from build123d import *

# Parameters (mm, degrees)
BOSS_EXTRUDE1_DEPTH = 14.2
BOSS_EXTRUDE2_DEPTH = 2.8
SKETCH3_R           = 1.7
CUT_EXTRUDE2_DEPTH  = 70.686512325


with BuildPart() as part:
    # Sketch1 → Boss-Extrude1 (new body)
    with BuildSketch(Plane(origin=(0, 0, 0), x_dir=(1, 0, 0), z_dir=(0, 1, 0))):
        Polygon((0, 21.05), (0, 31.1), (50, 31.1), (50, 21.05), (58, 21.05), (58, 10.05), (50, 10.05), (50, 0), (0, 0), (0, 10.05), (-8, 10.05), (-8, 21.05), align=None)
    extrude(amount=BOSS_EXTRUDE1_DEPTH)

    # Sketch2 → Boss-Extrude2 (add)
    with BuildSketch(Plane(origin=(0, 14.2, 0), x_dir=(1, 0, 0), z_dir=(0, 1, 0))):
        with BuildLine():
            Line((57.5, 31.1), (-7.5, 31.1))
            ThreePointArc((-7.5, 31.1), (-9.267766953, 30.367766953), (-10, 28.6))
            Line((-10, 28.6), (-10, 2.5))
            ThreePointArc((-10, 2.5), (-9.267766953, 0.732233047), (-7.5, 0))
            Line((-7.5, 0), (57.5, 0))
            ThreePointArc((57.5, 0), (59.267766953, 0.732233047), (60, 2.5))
            Line((60, 2.5), (60, 28.6))
            ThreePointArc((60, 28.6), (59.267766953, 30.367766953), (57.5, 31.1))
        make_face()
    extrude(amount=BOSS_EXTRUDE2_DEPTH)

    # Sketch3 → Cut-Extrude2 (cut, through all)
    with BuildSketch(Plane(origin=(0, 17, 0), x_dir=(1, 0, 0), z_dir=(0, 1, 0))):
        with Locations(Location((-6.8, 3.2, 0), (0, 0, 270))):
            Circle(SKETCH3_R)
        with Locations(Location((56.8, 3.2, 0), (0, 0, 270))):
            Circle(SKETCH3_R)
        with Locations(Location((56.8, 27.9, 0), (0, 0, 270))):
            Circle(SKETCH3_R)
        with Locations(Location((-6.8, 27.9, 0), (0, 0, 270))):
            Circle(SKETCH3_R)
    extrude(amount=-CUT_EXTRUDE2_DEPTH, mode=Mode.SUBTRACT)


solid = part.part
Work out the finished part from the listing and answer in its coordinate system (mm). A direction names the side the tool comes from. Give positions to 0.01 mm unless a question says otherwise; leave off trailing zeros. Order: outer loops, then holes, each group sorted by start corner. A loop starts at its lowest first (then second) coordinate and runs counter-clockwise, first axis right, second up. Notation, with made-up numbers: (22.25, 14.25) - (27.25, 14.25) arc R23 ccw to (27.25, 38.25) - close; hole circle Ø8 at (15, 45). An arc over 180 degrees is marked (long way). Answer as CSV lines item,"result". Start each with the question number.
Q1. Find the intervals of material crossed by L1, parallel to X at y = 16.4, z = -27.9; L2, parallel to X at y = 5, z = -2; L3, parallel to X at y = 14.25, z = -28.5, in increasing order. Write a range as [from, to].
Q2. For faces 1 (the face through (50, 7, -26)), 2 (the face through (0, 7, -5)), 3 (the face through (50, 7, -5)), 4 (the face through (-4, 7, -21.05)), determine the directions among +Z, -Z, +X, -X, +Y, -Y from which every point of the face is accessible in a straight line to the end or side of a thin tool.
Q3. The mould has two halves that part along Z. Classify faces 5 (the face through (59.287, 15.58, -30.348)), 6 (the face through (25, 8, 0)), 7 (the face through (-5.65, 15.62, -4.45)): +Z half, -Z half, draft (parallel to the pull), parting line (faces both ways), or undercut.
Q4. The part is cut by section B-B (z = -3.2). Write down the section's boundary in (x, y), then the cut area to 3 significant figures.
Q5. The part is cut by section C-C (y = 1.25). Write down the section's boundary in (x, z), then the cut area to 3 significant figures.
Q6. The part is cut by section D-D (z = -22). Write down the section's boundary in (x, y).
Q7. The part is cut by section A-A (x = -6.8). Write down the section's boundary in (y, z).
Q8. Given pin 1 Ø5 at (y, z) = (5, -3) entering from -X; pin 2 Ø5.5 at (y, z) = (7, -14) entering from -X; pin 3 Ø9 at (y, z) = (9.5, -16) entering from +X; pin 4 Ø2 at (x, z) = (-6.8, -27.9) entering from -Y, each flat-ended and moving along its own axis, determine where each tip first touches the part or whether it passes through.
Check result:
1,L1,"x = [-10, -8.5], [-5.1, 55.1], [58.5, 60]"
1,L2,"x = [0, 50]"
1,L3,"x = [-10, -8.39], [-5.21, 55.21], [58.39, 60]"
2,face 1,"-Z, +X, -Y"
2,face 2,"+Z, -X, -Y"
2,face 3,"+Z, +X, -Y"
2,face 4,"-Z, -X, -Y"
3,face 5,"-Z half"
3,face 6,"+Z half"
3,face 7,"undercut"
4,outline,"(-10, 14.2) - (-8.5, 14.2) - (-8.5, 17) - (-10, 17) - close; (-5.1, 14.2) - (0, 14.2) - (0, 0) - (50, 0) - (50, 14.2) - (55.1, 14.2) - (55.1, 17) - (-5.1, 17) - close; (58.5, 14.2) - (60, 14.2) - (60, 17) - (58.5, 17) - close"
4,area,"887 mm²"
5,outline,"(-8, -21.05) - (0, -21.05) - (0, -31.1) - (50, -31.1) - (50, -21.05) - (58, -21.05) - (58, -10.05) - (50, -10.05) - (50, 0) - (0, 0) - (0, -10.05) - (-8, -10.05) - close"
5,area,"1,730 mm²"
6,outline,"(-10, 14.2) - (0, 14.2) - (0, 0) - (50, 0) - (50, 14.2) - (60, 14.2) - (60, 17) - (-10, 17) - close"
7,outline,"(0, -21.05) - (14.2, -21.05) - (14.2, -26.2) - (17, -26.2) - (17, -4.9) - (14.2, -4.9) - (14.2, -10.05) - (0, -10.05) - close; (14.2, -31.1) - (17, -31.1) - (17, -29.6) - (14.2, -29.6) - close; (14.2, -1.5) - (17, -1.5) - (17, 0) - (14.2, 0) - close"
8,pin 1,"stops at x = 0"
8,pin 2,"stops at x = -8"
8,pin 3,"stops at x = 58"
8,pin 4,"passes through"
